Build history of the part. All positions in model axes, mm. A direction names the side the tool comes from. Give positions to 0.01 mm unless a question says otherwise; leave off trailing zeros. Loops run counter-clockwise (first coordinate to the right, second up) from the corner with the lowest first, then second, coordinate; pieces in that order, holes last.
1) Band-saw the part on D-D on z = 22. List the corners of the cut face in (x, y).
2) Band-saw the part on A-A on z = -20. List the corners of the cut face in (x, y), then the cut area to 3 significant figures.
3) 3-axis set-ups, long thin cutter, end or side, ignore diameter. For faces 5 (the cylindrical face through (32.5, 11.74, 37.45)), 6 (the cylindrical face through (30, 18, 32)), 7 (the flat face through (-33, 10.75, 22)), 8 (the flat face through (26, 12, 38.5)), 9 (the flat face through (12, 12, 34)): which of +Z, -Z, +X, -X, +Y, -Y reach the whole face in a straight line?
4) Two-plate mould, pull along Z, no slides. Class faces 1 (the cylindrical face through (27, 15, 31)), 2 (the flat face through (0, 18, 40)), 3 (the flat face through (18.6, 17.2, 37)), 4 (the flat face through (-33.5, 12, -30)): +Z half, -Z half, draft (parallel to the pull), parting line (faces both ways), or undercut.
5) Wall check: line 1 (X direction, y = 19.25, z = 35); line 2 (X direction, y = 12.35, z = -35); line 3 (X direction, y = 17, z = -2). Give the ranges that are in metal, low to high.
6) Flat gauge pins, fed straight in: P1, Ø0.6, axis at x = -27.5, y = 12, coming from the +Z side; P2, Ø1.5, axis at x = -19.5, z = -22, coming from the -Y side; P3, Ø1.5, axis at x = 10, y = 8, coming from the +Z side; P4, Ø1.8, axis at x = -30, z = 35, coming from the +Y side. Where does each tip first touch, or does it go through?
7) Band-saw the part on B-B on x = -17. List the corners of the cut face in (y, z).
8) Band-saw the part on C-C on x = 11. List the corners of the cut face in (y, z), then the cut area to 3 significant figures.
```python
from build123d import *

# Parameters (mm, degrees)
SKETCH1_W              = 70
SKETCH1_H              = 80
BOSS_EXTRUDE1_DEPTH    = 21.5
FILLET1_R              = 5
SHELL1_T               = 3
BOSS_EXTRUDE2_REACH    = 59.335
SKETCH3_R              = 5
SPLIT2_SURFACE_1_BACK  = 109.454
SPLIT2_SURFACE_1_DEPTH = 218.908
SPLIT2_SURFACE_2_BACK  = 109.454
SPLIT2_SURFACE_2_DEPTH = 218.908
SKETCH4_R              = 1
CUT_EXTRUDE1_DEPTH     = 58.334544561
SKETCH6_OUTSIDE_W      = 93.69
SKETCH6_OUTSIDE_H      = 103.69
CUT_EXTRUDE3_DEPTH     = 2
BOSS_EXTRUDE3_START    = 1.8
BOSS_EXTRUDE3_DEPTH    = 1.8
SKETCH8_R              = 5.5
CUT_EXTRUDE4_DEPTH     = 10
SKETCH9_R              = 5
SKETCH9_W              = 20
SKETCH9_H              = 12
CUT_EXTRUDE5_DEPTH     = 10
BOSS_EXTRUDE4_DEPTH    = 7.75
SKETCH5_R              = 3
CUT_EXTRUDE2_DEPTH     = 7.75
SKETCH12_W             = 31
SKETCH12_H             = 12
CUT_EXTRUDE6_DEPTH     = 10
BOSS_EXTRUDE5_DEPTH    = 5


with BuildPart() as part:
    # Sketch1 → Boss-Extrude1 (new body)
    with BuildSketch(Plane(origin=(0, 0, 0), x_dir=(1, 0, 0), z_dir=(0, 1, 0))):
        Rectangle(SKETCH1_W, SKETCH1_H)
    extrude(amount=BOSS_EXTRUDE1_DEPTH)

    # Fillet1
    fillet1_edges = [part.edges().sort_by_distance(p)[0] for p in [
        (-35, 10.75, -40),
        (35, 10.75, -40),
        (35, 10.75, 40),
        (-35, 10.75, 40),
    ]]
    fillet(fillet1_edges, radius=FILLET1_R)

    # Shell1 (no face opened: a closed hollow body)
    add(offset(amount=-SHELL1_T, mode=Mode.PRIVATE), mode=Mode.SUBTRACT)

    # Sketch3 → Boss-Extrude2 (add, up to next)
    with BuildSketch(Plane(origin=(0, 21.5, 0), x_dir=(1, 0, 0), z_dir=(0, 1, 0)), mode=Mode.PRIVATE) as boss_extrude2_sk1:
        with Locations((-30, 35)):
            Circle(SKETCH3_R)
    boss_extrude2_tool1 = extrude(boss_extrude2_sk1.sketch, amount=-BOSS_EXTRUDE2_REACH, mode=Mode.PRIVATE) - part.part
    # Sketch3 → Boss-Extrude2 (add, up to next)
    with BuildSketch(Plane(origin=(0, 21.5, 0), x_dir=(1, 0, 0), z_dir=(0, 1, 0)), mode=Mode.PRIVATE) as boss_extrude2_sk2:
        with Locations((30, 35)):
            Circle(SKETCH3_R)
    boss_extrude2_tool2 = extrude(boss_extrude2_sk2.sketch, amount=-BOSS_EXTRUDE2_REACH, mode=Mode.PRIVATE) - part.part
    # Sketch3 → Boss-Extrude2 (add, up to next)
    with BuildSketch(Plane(origin=(0, 21.5, 0), x_dir=(1, 0, 0), z_dir=(0, 1, 0)), mode=Mode.PRIVATE) as boss_extrude2_sk3:
        with Locations((30, -35)):
            Circle(SKETCH3_R)
    boss_extrude2_tool3 = extrude(boss_extrude2_sk3.sketch, amount=-BOSS_EXTRUDE2_REACH, mode=Mode.PRIVATE) - part.part
    # Sketch3 → Boss-Extrude2 (add, up to next)
    with BuildSketch(Plane(origin=(0, 21.5, 0), x_dir=(1, 0, 0), z_dir=(0, 1, 0)), mode=Mode.PRIVATE) as boss_extrude2_sk4:
        with Locations((-30, -35)):
            Circle(SKETCH3_R)
    boss_extrude2_tool4 = extrude(boss_extrude2_sk4.sketch, amount=-BOSS_EXTRUDE2_REACH, mode=Mode.PRIVATE) - part.part
    add(boss_extrude2_tool1.solids().sort_by_distance((-30, 21.5, -35))[0])
    add(boss_extrude2_tool2.solids().sort_by_distance((30, 21.5, -35))[0])
    add(boss_extrude2_tool3.solids().sort_by_distance((30, 21.5, 35))[0])
    add(boss_extrude2_tool4.solids().sort_by_distance((-30, 21.5, 35))[0])


with BuildPart() as body_2:
    # Split2: the piece behind the surface
    add(part.part)
    # Split2 surface: a surface, the sketch's curves swept straight by 218.908 mm
    with BuildLine(Plane(origin=(0, 0, 0), x_dir=(0, 0, -1), z_dir=(1, 0, 0)).offset(-SPLIT2_SURFACE_1_BACK), mode=Mode.PRIVATE) as split2_surface_1_path:
        Line((-40, 10.75), (51.562362236, 10.75))
    split2_surface_1 = Shell.extrude(split2_surface_1_path.wire(), (1 * SPLIT2_SURFACE_1_DEPTH, 0 * SPLIT2_SURFACE_1_DEPTH, 0 * SPLIT2_SURFACE_1_DEPTH))
    split(bisect_by=split2_surface_1, keep=Keep.BOTTOM)


with BuildPart() as part_1:
    add(part.part)

    # Split2: split by a surface, the side it looks to stays
    # Split2 surface: a surface, the sketch's curves swept straight by 218.908 mm
    with BuildLine(Plane(origin=(0, 0, 0), x_dir=(0, 0, -1), z_dir=(1, 0, 0)).offset(-SPLIT2_SURFACE_2_BACK), mode=Mode.PRIVATE) as split2_surface_2_path:
        Line((-40, 10.75), (51.562362236, 10.75))
    split2_surface_2 = Shell.extrude(split2_surface_2_path.wire(), (1 * SPLIT2_SURFACE_2_DEPTH, 0 * SPLIT2_SURFACE_2_DEPTH, 0 * SPLIT2_SURFACE_2_DEPTH))
    split(bisect_by=split2_surface_2, keep=Keep.TOP)


with BuildPart() as cut_extrude1_tool:
    # Sketch4 → Cut-Extrude1 (new, through all)
    with BuildSketch(Plane(origin=(0, 21.5, 0), x_dir=(1, 0, 0), z_dir=(0, 1, 0))):
        with Locations(Location((-30, 35, 0), (0, 0, 270))):
            Circle(SKETCH4_R)
        with Locations(Location((30, 35, 0), (0, 0, 270))):
            Circle(SKETCH4_R)
        with Locations(Location((30, -35, 0), (0, 0, 270))):
            Circle(SKETCH4_R)
        with Locations(Location((-30, -35, 0), (0, 0, 270))):
            Circle(SKETCH4_R)
    extrude(amount=-CUT_EXTRUDE1_DEPTH)


with BuildPart() as part_2:
    add(part_1.part)

    # Cut-Extrude1: cut by cut_extrude1_tool
    add(cut_extrude1_tool.part, mode=Mode.SUBTRACT)

    # Sketch6 outside → Cut-Extrude3 (cut)
    with BuildSketch(Plane.XZ.offset(-10.75)):
        Rectangle(SKETCH6_OUTSIDE_W, SKETCH6_OUTSIDE_H)
        with BuildLine():
            Line((-30, -38.5), (30, -38.5))
            ThreePointArc((30, -38.5), (32.474873734, -37.474873734), (33.5, -35))
            Line((33.5, -35), (33.5, 35))
            ThreePointArc((33.5, 35), (32.474873734, 37.474873734), (30, 38.5))
            Line((30, 38.5), (-30, 38.5))
            ThreePointArc((-30, 38.5), (-32.474873734, 37.474873734), (-33.5, 35))
            Line((-33.5, 35), (-33.5, -35))
            ThreePointArc((-33.5, -35), (-32.474873734, -37.474873734), (-30, -38.5))
        make_face(mode=Mode.SUBTRACT)
    extrude(amount=-CUT_EXTRUDE3_DEPTH, mode=Mode.SUBTRACT)


with BuildPart() as body_2_1:
    add(body_2.part)

    # Cut-Extrude1: cut by cut_extrude1_tool
    add(cut_extrude1_tool.part, mode=Mode.SUBTRACT)

    # Sketch7 → Boss-Extrude3 (add)
    with BuildSketch(Plane(origin=(0, 10.75, 0), x_dir=(1, 0, 0), z_dir=(0, 1, 0)).offset(BOSS_EXTRUDE3_START)):
        with BuildLine():
            Line((-30, 40), (30, 40))
            ThreePointArc((30, 40), (33.535533906, 38.535533906), (35, 35))
            Line((35, 35), (35, -35))
            ThreePointArc((35, -35), (33.535533906, -38.535533906), (30, -40))
            Line((30, -40), (-30, -40))
            ThreePointArc((-30, -40), (-33.535533906, -38.535533906), (-35, -35))
            Line((-35, -35), (-35, 35))
            ThreePointArc((-35, 35), (-33.535533906, 38.535533906), (-30, 40))
        make_face()
        with BuildLine():
            Line((30, 38.7), (-30, 38.7))
            ThreePointArc((-30, 38.7), (-32.61629509, 37.61629509), (-33.7, 35))
            Line((-33.7, 35), (-33.7, -35))
            ThreePointArc((-33.7, -35), (-32.61629509, -37.61629509), (-30, -38.7))
            Line((-30, -38.7), (30, -38.7))
            ThreePointArc((30, -38.7), (32.61629509, -37.61629509), (33.7, -35))
            Line((33.7, -35), (33.7, 35))
            ThreePointArc((33.7, 35), (32.61629509, 37.61629509), (30, 38.7))
        make_face(mode=Mode.SUBTRACT)
    extrude(amount=-BOSS_EXTRUDE3_DEPTH)


with BuildPart() as cut_extrude4_tool:
    # Sketch8 → Cut-Extrude4 (new body)
    with BuildSketch(Plane.ZY.offset(35)):
        with Locations((-20, 12.05)):
            Circle(SKETCH8_R)
    extrude(amount=-CUT_EXTRUDE4_DEPTH)


with BuildPart() as part_3:
    add(part_2.part)

    # Cut-Extrude4: cut by cut_extrude4_tool
    add(cut_extrude4_tool.part, mode=Mode.SUBTRACT)


with BuildPart() as body_2_2:
    add(body_2_1.part)

    # Cut-Extrude4: cut by cut_extrude4_tool
    add(cut_extrude4_tool.part, mode=Mode.SUBTRACT)


with BuildPart() as cut_extrude5_tool:
    # Sketch9 → Cut-Extrude5 (new body)
    with BuildSketch(Plane.XY.offset(40)):
        with Locations((18, 12.05)):
            Circle(SKETCH9_R)
        with Locations((-10, 10.75)):
            Rectangle(SKETCH9_W, SKETCH9_H)
    extrude(amount=-CUT_EXTRUDE5_DEPTH)


with BuildPart() as part_4:
    add(part_3.part)

    # Cut-Extrude5: cut by cut_extrude5_tool
    add(cut_extrude5_tool.part, mode=Mode.SUBTRACT)

    # Sketch11 → Boss-Extrude4 (add)
    with BuildSketch(Plane.XZ.offset(-18.5)):
        Polygon((-28, 38.5), (12, 38.5), (12, 32), (7.5, 32), (7.5, 35), (9, 35), (9, 37), (-25, 37), (-25, 35), (-23.5, 35), (-23.5, 32), (-28, 32), align=None)
    extrude(amount=BOSS_EXTRUDE4_DEPTH)

    # Sketch5 → Cut-Extrude2 (cut)
    with BuildSketch(Plane(origin=(0, 21.5, 0), x_dir=(1, 0, 0), z_dir=(0, 1, 0))):
        with Locations(Location((-30, 35, 0), (0, 0, 270))):
            Circle(SKETCH5_R)
        with Locations(Location((30, 35, 0), (0, 0, 270))):
            Circle(SKETCH5_R)
        with Locations(Location((30, -35, 0), (0, 0, 270))):
            Circle(SKETCH5_R)
        with Locations(Location((-30, -35, 0), (0, 0, 270))):
            Circle(SKETCH5_R)
    extrude(amount=-CUT_EXTRUDE2_DEPTH, mode=Mode.SUBTRACT)


with BuildPart() as body_2_3:
    add(body_2_2.part)

    # Cut-Extrude5: cut by cut_extrude5_tool
    add(cut_extrude5_tool.part, mode=Mode.SUBTRACT)


with BuildPart() as cut_extrude6_tool:
    # Sketch12 → Cut-Extrude6 (new body)
    with BuildSketch(Plane(origin=(0, 0, 37), x_dir=(-1, 0, 0), z_dir=(0, 0, -1))):
        with Locations((8, 10.75)):
            Rectangle(SKETCH12_W, SKETCH12_H)
    extrude(amount=-CUT_EXTRUDE6_DEPTH)


with BuildPart() as part_5:
    add(part_4.part)

    # Cut-Extrude6: cut by cut_extrude6_tool
    add(cut_extrude6_tool.part, mode=Mode.SUBTRACT)

    # Sketch14 → Boss-Extrude5 (add)
    with BuildSketch(Plane.XZ.offset(-10.75)):
        Polygon((12, 36.8), (9, 36.8), (9, 35), (7.5, 35), (7.5, 32), (12, 32), align=None)
    extrude(amount=BOSS_EXTRUDE5_DEPTH)


with BuildPart() as body_2_4:
    add(body_2_3.part)

    # Cut-Extrude6: cut by cut_extrude6_tool
    add(cut_extrude6_tool.part, mode=Mode.SUBTRACT)


solid = part_5.part
```
Findings below:
1. outline: (-35, 12.75) - (-33.5, 12.75) - (-33.5, 10.75) - (-32, 10.75) - (-32, 18.5) - (32, 18.5) - (32, 10.75) - (33.5, 10.75) - (33.5, 12.75) - (35, 12.75) - (35, 21.5) - (-35, 21.5) - close
2. outline: (-35, 17.55) - (-32, 17.55) - (-32, 18.5) - (32, 18.5) - (32, 10.75) - (33.5, 10.75) - (33.5, 12.75) - (35, 12.75) - (35, 21.5) - (-35, 21.5) - close
2. area: 233 mm2
3. face 5: +Z, +X, -Y
3. face 6: +Y
3. face 7: +Z, -Z, -X, -Y
3. face 8: +Z, +X, -X, -Y
3. face 9: -Y
4. face 1: undercut
4. face 2: +Z half
4. face 3: undercut
4. face 4: draft
5. line 1: x = -35 to -33, -27 to 27, 33 to 35
5. line 2: x = -33.5 to -31, -29 to -25, 25 to 29, 31 to 33.5
5. line 3: x = -35 to -32, 32 to 35
6. P1: stops at z = 38.5
6. P2: stops at y = 18.5
6. P3: stops at z = 36.8
6. P4: passes through
7. outline: (10.75, -38.5) - (12.75, -38.5) - (12.75, -40) - (21.5, -40) - (21.5, 40) - (16.75, 40) - (16.75, 37) - (18.5, 37) - (18.5, -37) - (10.75, -37) - close
8. outline: (5.75, 32) - (18.5, 32) - (18.5, -37) - (10.75, -37) - (10.75, -38.5) - (12.75, -38.5) - (12.75, -40) - (21.5, -40) - (21.5, 40) - (12.75, 40) - (12.75, 38.5) - (10.75, 38.5) - (10.75, 36.8) - (5.75, 36.8) - close
8. area: 343 mm2
